```python
from build123d import *

# Parameters (mm, degrees)
SKETCH024_W                   = 95
SKETCH024_H                   = 82
PAD006_DEPTH                  = 3
SKETCH025_W                   = 11
SKETCH025_H                   = 3
SKETCH025_W_2                 = 16
SKETCH025_W_3                 = 3
SKETCH025_H_2                 = 11
SKETCH025_H_3                 = 14.5
POCKET018_DEPTH               = 254.062745
POCKET019_DEPTH               = 254.062745
POCKET019_MIRRORED022_2_DEPTH = 254.062745
POCKET020_DEPTH               = 3.001
SKETCH025_MIRRORED024_2_W     = 11
SKETCH025_MIRRORED024_2_H     = 3
SKETCH025_MIRRORED024_2_W_2   = 16
SKETCH025_MIRRORED024_2_W_3   = 3
SKETCH025_MIRRORED024_2_H_2   = 11
SKETCH025_MIRRORED024_2_H_3   = 14.5
POCKET018_MIRRORED024_2_DEPTH = 254.062745
SKETCH028_W                   = 4
SKETCH028_H                   = 2.5
POCKET021_DEPTH               = 3.001


with BuildPart() as part:
    # Sketch024 → Pad006 (new body)
    with BuildSketch(Plane.YZ):
        Rectangle(SKETCH024_W, SKETCH024_H)
    extrude(amount=PAD006_DEPTH)

    # Sketch025 → Pocket018 (cut, through all)
    with BuildSketch(Plane.YZ):
        with Locations((0, 39.5)):
            Rectangle(SKETCH025_W, SKETCH025_H)
        with Locations((33.5, 39.5)):
            Rectangle(SKETCH025_W_2, SKETCH025_H)
        with Locations((46, 0)):
            Rectangle(SKETCH025_W_3, SKETCH025_H_2)
        with Locations((46, 30.75)):
            Rectangle(SKETCH025_W_3, SKETCH025_H_3)
    pocket018 = extrude(amount=POCKET018_DEPTH, mode=Mode.SUBTRACT)

    # Sketch026 → Pocket019 (cut, through all)
    with BuildSketch(Plane.YZ):
        Polygon((-32.25, 41), (-32.25, 32), (-31, 32), (-31, 30), (-32.25, 30), (-32.25, 27), (-34.75, 27), (-34.75, 30), (-36, 30), (-36, 32), (-34.75, 32), (-34.75, 41), align=None)
    pocket019 = extrude(amount=POCKET019_DEPTH, mode=Mode.SUBTRACT)

    # Sketch026 Mirrored022 2 → Pocket019 Mirrored022 2 (cut, through all)
    with BuildSketch(Plane(origin=(0, 0, 0), x_dir=(0, -1, 0), z_dir=(-1, 0, 0))):
        Polygon((-32.25, 41), (-32.25, 32), (-31, 32), (-31, 30), (-32.25, 30), (-32.25, 27), (-34.75, 27), (-34.75, 30), (-36, 30), (-36, 32), (-34.75, 32), (-34.75, 41), align=None)
    pocket019_mirrored022_2 = extrude(amount=-POCKET019_MIRRORED022_2_DEPTH, mode=Mode.SUBTRACT)

    # Mirrored023: Pocket019, Pocket019 Mirrored022 2 across Sketch026 H_Axis
    add(pocket019.mirror(Plane.XY), mode=Mode.SUBTRACT)
    add(pocket019_mirrored022_2.mirror(Plane.XY), mode=Mode.SUBTRACT)

    # Sketch027 → Pocket020 (cut, through all)
    with BuildSketch(Plane.YZ):
        with BuildLine():
            Line((-6, 30), (6, 30))
            ThreePointArc((9, 27), (8.12132, 29.12132), (6, 30))
            Line((9, 27), (9, 8))
            ThreePointArc((6, 5), (8.12132, 5.87868), (9, 8))
            Line((6, 5), (-6, 5))
            ThreePointArc((-9, 8), (-8.12132, 5.87868), (-6, 5))
            Line((-9, 8), (-9, 27))
            ThreePointArc((-6, 30), (-8.12132, 29.12132), (-9, 27))
        make_face()
    extrude(amount=POCKET020_DEPTH, mode=Mode.SUBTRACT)

    # Sketch025 Mirrored024 2 → Pocket018 Mirrored024 2 (cut, through all)
    with BuildSketch(Plane(origin=(0, 0, 0), x_dir=(0, -1, 0), z_dir=(-1, 0, 0))):
        with Locations((0, 39.5)):
            Rectangle(SKETCH025_MIRRORED024_2_W, SKETCH025_MIRRORED024_2_H)
        with Locations((33.5, 39.5)):
            Rectangle(SKETCH025_MIRRORED024_2_W_2, SKETCH025_MIRRORED024_2_H)
        with Locations((46, 0)):
            Rectangle(SKETCH025_MIRRORED024_2_W_3, SKETCH025_MIRRORED024_2_H_2)
        with Locations((46, 30.75)):
            Rectangle(SKETCH025_MIRRORED024_2_W_3, SKETCH025_MIRRORED024_2_H_3)
    pocket018_mirrored024_2 = extrude(amount=-POCKET018_MIRRORED024_2_DEPTH, mode=Mode.SUBTRACT)

    # Mirrored025: Pocket018, Pocket018 Mirrored024 2 across Sketch025 H_Axis
    add(pocket018.mirror(Plane.XY), mode=Mode.SUBTRACT)
    add(pocket018_mirrored024_2.mirror(Plane.XY), mode=Mode.SUBTRACT)

    # Sketch028 → Pocket021 (cut, through all)
    with BuildSketch(Plane.YZ):
        with Locations((-45.5, -14.5)):
            Rectangle(SKETCH028_W, SKETCH028_H)
        with Locations((45.5, -14.5)):
            Rectangle(SKETCH028_W, SKETCH028_H)
        with Locations((45.5, 14.5)):
            Rectangle(SKETCH028_W, SKETCH028_H)
    extrude(amount=POCKET021_DEPTH, mode=Mode.SUBTRACT)


with BuildPart() as part_1:
    # Body006 placement: moved
    add(part.part.moved(Location((-60, 0, 0))))


solid = part_1.part
```
Could you check a few things on this model? Use its own coordinates, in mm. A direction names the side the tool comes from. Give positions to 0.01 mm unless a question says otherwise; leave off trailing zeros. Write each loop counter-clockwise with the first axis right and the second up, starting at its lowest first coordinate (ties: lowest second). Pieces come first, ordered by that corner, then holes. Notation, with made-up numbers: (-26.5, 74.25) - (3.5, 74.25) arc R23 ccw to (3.5, 91.25) - close; hole circle Ø8 at (-7.75, -14.75). An arc over 180 degrees is marked (long way). One line per item, written item: value. Start each with the question number.
Item 1: Imagine slicing it at B-B, the plane z = 1. List the corners of the cut face in (x, y) for me, and give its area (3 significant figures).
Item 2: I'm going to push flat-ended pins straight in: pin 1 (1.5 mm diameter, centred on x = -58, y = -37.5, fed in from +Z); pin 2 (1 mm diameter, centred on x = -58.5, z = -31.5, fed in from -Y); pin 3 (1.2 mm diameter, centred on x = -59, y = 33, fed in from -Z); pin 4 (1 mm diameter, centred on x = -58, z = 15.5, fed in from +Y). Where does each tip first touch, or does it pass through?
Item 3: If we mould it in two halves opening along Y, with no side actions, what happens to faces 1 (the face through (-59, 44.5, 0)), 2 (the face through (-59, 46, -38)), 3 (the face through (-59, 34.75, -28))? For each: +Y half, -Y half, draft (parallel to the pull), parting line (faces both ways), or undercut.
Item 4: Imagine slicing it at A-A, the plane y = -4. List the corners of the cut face in (x, z) for me, and give its area (3 significant figures).
Item 5: Imagine slicing it at C-C, the plane y = 39. List the corners of the cut face in (x, z) for me.
Item 6: Please list where these lines run through material, in increasing order: line 1 (Z direction, x = -58.25, y = -32); line 2 (Y direction, x = -58.75, z = 26.5); line 3 (Z direction, x = -58.4, y = -1). Write a range as from..to.
Item 7: Which directions (+Z, -Z, +X, -X, +Y, -Y) give clear straight access to the entire face, cutting with the end or side of a thin tool? Please do faces 4 (the face through (-59, 45, -15.75)), 5 (the face through (-58.52, -8.1, 29.14)), 6 (the face through (-59, -5.5, -39)), 7 (the face through (-59, -46, -5.5)).
Geometry says:
1. outline: (-60, -44.5) - (-57, -44.5) - (-57, 44.5) - (-60, 44.5) - close
1. area: 267 mm^2
2. pin 1: z = 38
2. pin 2: y = -44.5
2. pin 3: z = -27
2. pin 4: y = 47.5
3. face 1: +Y half
3. face 2: draft
3. face 3: undercut
4. outline: (-60, -38) - (-57, -38) - (-57, 5) - (-60, 5) - close; (-60, 30) - (-57, 30) - (-57, 38) - (-60, 38) - close
4. area: 153 mm^2
5. outline: (-60, -38) - (-57, -38) - (-57, 38) - (-60, 38) - close
6. line 1: -38..-32, -30..30, 32..38
6. line 2: -44.5..-9, 9..44.5
6. line 3: -38..5, 30..38
7. face 4: +X, -X, +Y
7. face 5: +X, -X
7. face 6: -Z, +X, -X
7. face 7: +X, -X, -Y
